Geometry: see drawing. Coordinates: mm, zero at the bounding-box minimum. A direction names the side the tool comes from. Coordinates: 2 decimals unless noted, no trailing zeros. Order: outer loops, then holes, each group sorted by start corner. A loop starts at its lowest first (then second) coordinate and runs counter-clockwise, first axis right, second up. Notation, with made-up numbers: (44.5, 10.5) -> (77.5, 10.5) arc R16 cw to (77.5, 22.5) -> close; hole circle Ø3 at (49.5, -19). An arc over 180 degrees is marked (long way). Use one line per item in the form item = value.
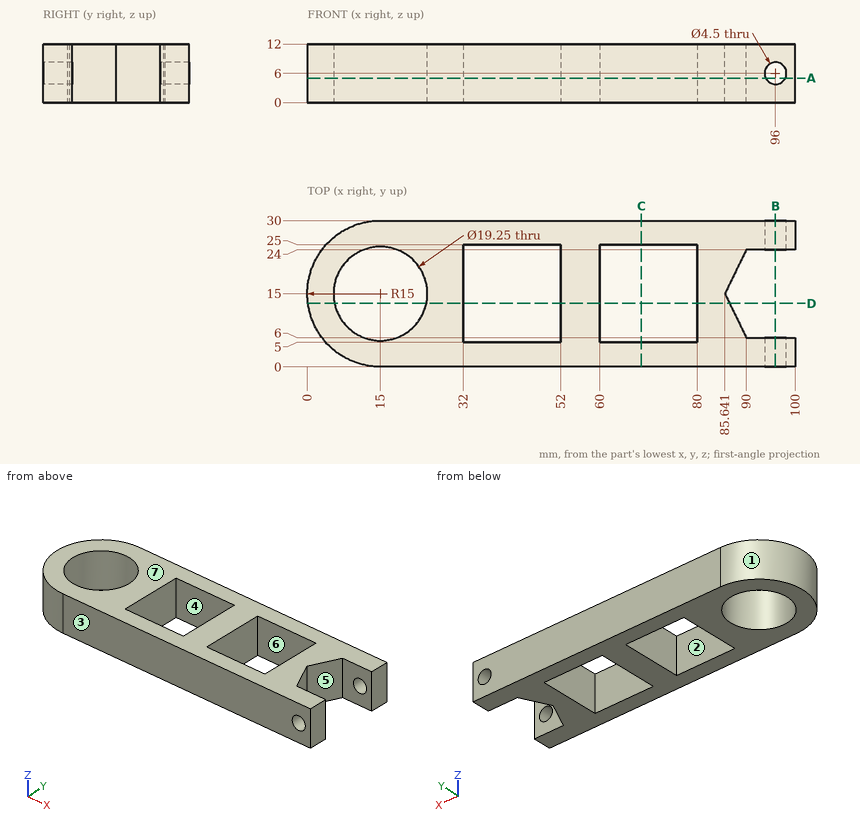
1) Pull-direction query (Y, two-part tool) for the marked faces 1, 2, 3 and 4; classes: released by +Y, released by -Y, zero draft, split by the parting line, or undercut.
Results found:
face_1 = split by the parting line
face_2 = undercut
face_3 = released by -Y
face_4 = undercut
2) Section B-B, the plane x = 96. Output: boundary loops of the cut face in (y, z), and give its area (3 significant figures).
Results found:
outline = (0, 0) -> (6, 0) -> (6, 3.75) -> (0, 3.75) -> close; (0, 8.25) -> (6, 8.25) -> (6, 12) -> (0, 12) -> close; (24, 0) -> (30, 0) -> (30, 3.75) -> (24, 3.75) -> close; (24, 8.25) -> (30, 8.25) -> (30, 12) -> (24, 12) -> close
area = 90.0 mm2
3) Access query for the marked faces 5, 6 and 7. Directions: +Z, -Z, +X, -X, +Y, -Y. A direction counts if a zero-diameter tool reaches every point of the face in a straight line with its end or side. Return the directions, or none.
Results found:
face_5 = +Z, -Z, +X
face_6 = +Z, -Z
face_7 = +Z, +X, -X, +Y, -Y
4) Section A-A, the plane z = 5. Give the number of separate pieces and of enclosed holes in the cut face, and give its area (3 significant figures).
Results found:
separate_pieces = 3
enclosed_holes = 3
area = 1,540 mm2
5) Section C-C, the plane x = 68.5. Output: boundary loops of the cut face in (y, z), and give its area (3 significant figures).
Results found:
outline = (0, 0) -> (5, 0) -> (5, 12) -> (0, 12) -> close; (25, 0) -> (30, 0) -> (30, 12) -> (25, 12) -> close
area = 120 mm2
6) Contact query for flat-ended pins moving along their axis: P1, Ø3, axis at y = 19.5, z = 9.5, coming from the -X side; P2, Ø6, axis at x = 47, z = 8, coming from the -Y side; P3, Ø6, axis at y = 24.5, z = 5.5, coming from the -X side; P4, Ø3.5, axis at y = 18.5, z = 7, coming from the +X side. Output: stop coordinate, or through.
Results found:
P1 = 0.3
P2 = 0
P3 = 1.48
P4 = 88.18
7) Section D-D, the plane y = 13. Output: boundary loops of the cut face in (x, z) (3 decimals), and give its area (3 significant figures).
Results found:
outline = (0.134, 0) -> (5.585, 0) -> (5.585, 12) -> (0.134, 12) -> close; (24.415, 0) -> (32, 0) -> (32, 12) -> (24.415, 12) -> close; (52, 0) -> (60, 0) -> (60, 12) -> (52, 12) -> close; (80, 0) -> (86.61, 0) -> (86.61, 12) -> (80, 12) -> close
area = 332 mm2
8) Material intervals for probe 1 along Y at (x, z) = (96, 10.25); probe 2 along Y at (x, z) = (15, 6) (3 decimals); probe 3 along Z at (x, y) = (96, 3.85), sorted ascending. Write a range as from..to.
Results found:
probe_1 = 0..6, 24..30
probe_2 = 0..5.375, 24.625..30
probe_3 = 0..3.75, 8.25..12
